Autodesk Inventor part; units mm, degrees
ref_plane "YZ Plane" through (0, 0, 0) normal (1, 0, 0) x (0, 1, 0)
ref_plane "XZ Plane" through (0, 0, 0) normal (0, 1, 0) x (-1, 0, 0)
ref_plane "XY Plane" through (0, 0, 0) normal (0, 0, 1) x (1, 0, 0)
sketch "Sketch1" plane through (0, 0, 0) normal (0, 0, 1) x (1, 0, 0)
  line L0 (0, 0) -> (30, 0)
  line L1 (30, 0) -> (30, 3)
  line L2 (30, 3) -> (3, 3)
  line L3 (3, 3) -> (3, 30)
  line L4 (3, 30) -> (0, 30)
  line L5 (0, 0) -> (-30, 0)
  line L6 (-30, 0) -> (-30, 3)
  line L7 (-30, 3) -> (0, 3)
  line L8 (0, 3) -> (0, 30)
  dimension "d0" = 3
  dimension "d2" = 30
  dimension "d5" = 3
extrude "Extrusion1" add sketch "Sketch1" along normal blind 1800
sketch "Sketch2" plane through (3, 3, 1800) normal (0, 1, 0) x (1, 0, 0)
  line L0 (-3, 0) -> (-33, 0)
  line L1 (-3, 1800) -> (-3, 0)
  line L2 (0, 1800) -> (0, 0)
  line L3 (27, 0) -> (0, 0)
  point P0 (15, 15)
  point P1 (-18, 15)
  point P2 (-18, 465)
  point P3 (15, 465)
  point P4 (15, 915)
  point P5 (-18, 915)
  point P6 (-18, 1365)
  point P7 (15, 1365)
  dimension "d8" = 15
  dimension "d9" = 15
  dimension "d10" = 15
  dimension "d11" = 15
  dimension "d12" = 450
  dimension "d13" = 450
  dimension "d14" = 15
  dimension "d15" = 15
  dimension "d16" = 450
  dimension "d17" = 450
  dimension "d18" = 15
  dimension "d19" = 15
  dimension "d20" = 450
  dimension "d21" = 450
  dimension "d22" = 15
  dimension "d23" = 15
hole "Hole1" at (18, 3, 1785) at (-15, 3, 1785) at (-15, 3, 1335) at (18, 3, 1335) at (18, 3, 885) at (-15, 3, 885) at (-15, 3, 435) at (18, 3, 435) direction (0, -1, 0) diameter 3.81 end through all
sketch "Sketch3" plane through (3, 30, 1800) normal (1, 0, 0) x (0, 0, -1)
  line L0 (0, -27) -> (0, 0)
  line L1 (1800, -27) -> (0, -27)
  point P0 (1800, -30)
  point P1 (15, -12)
  point P2 (465, -12)
  point P3 (915, -12)
  point P4 (1365, -12)
  dimension "d31" = 15
  dimension "d32" = 15
  dimension "d33" = 450
  dimension "d34" = 15
  dimension "d35" = 450
  dimension "d36" = 450
  dimension "d37" = 15
  dimension "d38" = 15
hole "Hole2" at (3, 18, 1785) at (3, 18, 1335) at (3, 18, 885) at (3, 18, 435) direction (-1, 0, 0) diameter 3.81 end through all
equation "\"d0\" = Thickness"
equation "\"d2\" = Width"
equation "\"d5\" = Thickness"
equation "\"d6\" = Height"
equation "\"Width\" = 30"
equation "\"Thickness\" = 3"
equation "\"Height\" = 1800"
equation "\"HoleDistance\" = 15"
properties part number "mid180"
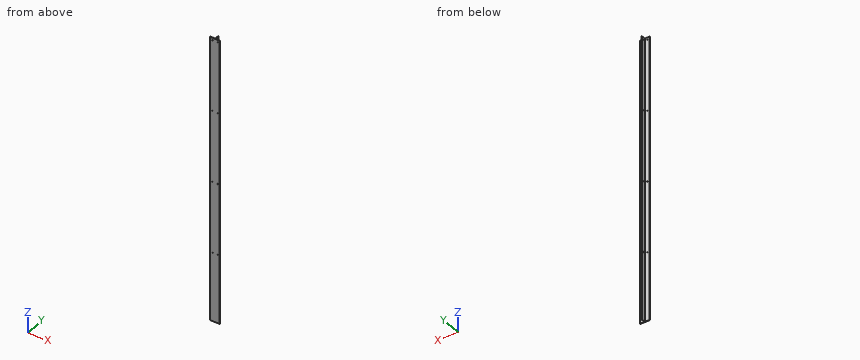
Geometry: final body of the model. Coordinates: model frame, mm. Coordinates: 2 decimals unless noted, no trailing zeros. Loops run counter-clockwise (first coordinate to the right, second up) from the corner with the lowest first, then second, coordinate; pieces in that order, holes last. Notation, with made-up numbers: (6, 32) -> (47, 32) arc R20 cw to (47, 65) -> close; hole circle Ø6 at (-26.75, 68.25). An arc over 180 degrees is marked (long way). Use a Markdown table: item, result. Add a question column.
(1) Pin query (flat end, axial travel): pin 1 Ø3.5 at (x, z) = (-15, 1335) entering from +Y; pin 2 Ø10 at (y, z) = (25, 245) entering from +X; pin 3 Ø6 at (y, z) = (18, 435) entering from -X; pin 4 Ø8 at (x, z) = (10, 971.5) entering from +Y. Return the tip coordinate at first contact, or that it passes through.
(2) Section query A-A, the plane z = 1595. Return loops of the section in (x, y), plus the area to 3 significant figures.
(3) Line query: line 1 along Z through (x, y) = (18, 2.25) (3 decimals); line 2 along X through (y, z) = (1.95, 435) (3 decimals); line 3 along Y through (x, z) = (1, 1335) (3 decimals). Output: solid intervals per line, ascending.
Answer:
| question | item | result |
|---|---|---|
| 1 | pin 1 | passes through |
| 1 | pin 2 | stops at x = 3 |
| 1 | pin 3 | stops at x = 0 |
| 1 | pin 4 | stops at y = 3 |
| 2 | outline | (-30, 0) -> (30, 0) -> (30, 3) -> (3, 3) -> (3, 30) -> (0, 30) -> (0, 3) -> (-30, 3) -> close |
| 2 | area | 261 mm^2 |
| 3 | line 1 | z = 0 to 433.095, 436.905 to 883.095, 886.905 to 1333.095, 1336.905 to 1783.095, 1786.905 to 1800 |
| 3 | line 2 | x = -30 to -16.905, -13.095 to 16.095, 19.905 to 30 |
| 3 | line 3 | y = 0 to 16.095, 19.905 to 30 |
